Geometry: final body of the model. Coordinates: model frame, mm. A direction names the side the tool comes from. Give positions to 0.01 mm unless a question says otherwise; leave off trailing zeros. Write each loop counter-clockwise with the first axis right and the second up, starting at its lowest first coordinate (ties: lowest second). Pieces come first, ordered by that corner, then holes. Notation, with made-up numbers: M 16,9 L 21,9 A6 cw 21,17 Z; hole C 64.5,84 d4. An arc over 180 degrees is marked long. Answer as a JSON object with one key per item and string values.
from build123d import *

# Parameters (mm, degrees)
EXTRUDE1_DEPTH = 9.525
EXTRUDE2_DEPTH = 6.35


with BuildPart() as part:
    # Sketch1 → Extrude1 (new body)
    with BuildSketch(Plane(origin=(0, 0, 0), x_dir=(1, 0, 0), z_dir=(0, 1, 0))):
        with BuildLine():
            Line((4.7752, 0), (82.475669818, 0))
            ThreePointArc((82.475669818, 0), (85.852246119, 1.398623698), (87.250869818, 4.7752))
            Line((87.250869818, 4.7752), (87.250869818, 46.540933005))
            ThreePointArc((87.250869818, 46.540933005), (85.852246119, 49.917509306), (82.475669818, 51.316133005))
            Line((82.475669818, 51.316133005), (4.7752, 51.316133005))
            ThreePointArc((4.7752, 51.316133005), (1.398623698, 49.917509306), (0, 46.540933005))
            Line((0, 46.540933005), (0, 4.7752))
            ThreePointArc((0, 4.7752), (1.398623698, 1.398623698), (4.7752, 0))
        make_face()
    extrude(amount=-EXTRUDE1_DEPTH)

    # Sketch2 → Extrude2 (cut)
    with BuildSketch(Plane(origin=(0, 0, 0), x_dir=(1, 0, 0), z_dir=(0, 1, 0))):
        with BuildLine():
            Line((3.175, 46.540933005), (3.175, 4.7752))
            ThreePointArc((3.175, 4.7752), (3.643687729, 3.643687729), (4.7752, 3.175))
            Line((4.7752, 3.175), (82.475669818, 3.175))
            ThreePointArc((82.475669818, 3.175), (83.607182089, 3.643687729), (84.075869818, 4.7752))
            Line((84.075869818, 4.7752), (84.075869818, 46.540933005))
            ThreePointArc((84.075869818, 46.540933005), (83.607182089, 47.672445276), (82.475669818, 48.141133005))
            Line((82.475669818, 48.141133005), (4.7752, 48.141133005))
            ThreePointArc((4.7752, 48.141133005), (3.643687729, 47.672445276), (3.175, 46.540933005))
        make_face()
    extrude(amount=-EXTRUDE2_DEPTH, mode=Mode.SUBTRACT)


solid = part.part
1) Cut plane B-B on x = 19.5. Return loops of the section in (y, z) (3 decimals).
Geometry check:
{"outline": "M -9.525,-51.316 L 0,-51.316 L 0,-48.141 L -6.35,-48.141 L -6.35,-3.175 L 0,-3.175 L 0,0 L -9.525,0 Z"}
2) Set-up query: faces 4 (the flat face through (43, -3, -3.175)), 5 (the cylindrical face through (85.815, -4.696, -1.362)). Return all of +Z, -Z, +X, -X, +Y, -Y with unobstructed straight access to the full face (end or side cutting, diameter ignored); none if empty.
Geometry check:
{"face 4": "+Y", "face 5": "+Z, +X, +Y, -Y"}
3) Contact query for flat-ended pins moving along their axis: P1, Ø8, axis at x = 23.5, z = -10, coming from the +Y side; P2, Ø22.5, axis at x = 30, z = -37, coming from the +Y side. Output: stop coordinate, or through.
Geometry check:
{"P1": "stops at y = -6.35", "P2": "stops at y = 0"}
4) Cut plane C-C on z = -39. Return loops of the section in (x, y) (3 decimals), and give its area (3 significant figures).
Geometry check:
{"outline": "M 0,-9.525 L 87.251,-9.525 L 87.251,0 L 84.076,0 L 84.076,-6.35 L 3.175,-6.35 L 3.175,0 L 0,0 Z", "area": "317 mm2"}
5) Line query: line 1 (Z direction, x = 59, y = -0.75) (3 decimals); line 2 (X direction, y = -3.5, z = -42) (3 decimals); line 3 (Y direction, x = 52, z = -39.5) (3 decimals). Output: solid intervals per line, ascending. Write a range as from..to.
Geometry check:
{"line 1": "z = -51.316..-48.141, -3.175..0", "line 2": "x = 0..3.175, 84.076..87.251", "line 3": "y = -9.525..-6.35"}
6) Cut plane A-A on y = -1.5. Return loops of the section in (x, z) (3 decimals), and give its area (3 significant figures).
Geometry check:
{"outline": "M 0,-46.541 A4.775 ccw 4.775,-51.316 L 82.476,-51.316 A4.775 ccw 87.251,-46.541 L 87.251,-4.775 A4.775 ccw 82.476,0 L 4.775,0 A4.775 ccw 0,-4.775 Z; hole M 3.175,-46.541 A1.6 ccw 4.775,-48.141 L 82.476,-48.141 A1.6 ccw 84.076,-46.541 L 84.076,-4.775 A1.6 ccw 82.476,-3.175 L 4.775,-3.175 A1.6 ccw 3.175,-4.775 Z", "area": "822 mm2"}
7) Pull-direction query (Z, two-part tool) for faces 1 (the flat face through (43, -5, 0)), 2 (the flat face through (43, -9.525, -26)), 3 (the flat face through (84.076, -3, -25)); classes: pulls with the +Z half, pulls with the -Z half, needs draft (parallel to the pull), parting line crosses it, or undercut.
Geometry check:
{"face 1": "pulls with the +Z half", "face 2": "needs draft", "face 3": "undercut"}
